```python
from build123d import *

# Parameters (mm, degrees)
SKETCH1_W           = 11
SKETCH1_H           = 70
SKETCH1_W_2         = 40
SKETCH1_H_2         = 18
BOSS_EXTRUDE1_DEPTH = 5
SKETCH3_W           = 23
SKETCH3_H           = 13
CUT_EXTRUDE2_DEPTH  = 57.868268832
SKETCH4_R           = 1.25
CUT_EXTRUDE3_DEPTH  = 57.868268832
SKETCH5_W           = 11
SKETCH5_H           = 75
BOSS_EXTRUDE2_DEPTH = 9
SKETCH6_W           = 3.5
SKETCH6_H           = 70
CUT_EXTRUDE4_DEPTH  = 59.352377844
SKETCH7_R           = 2
CUT_EXTRUDE5_DEPTH  = 61.458663564
RIB2_REACH          = 80.873
SKETCH8_WALL_W      = 176.81268046
SKETCH8_WALL_H      = 5
RIB4_REACH          = 80.873
SKETCH9_WALL_W      = 176.81268046
SKETCH9_WALL_H      = 5
RIB8_REACH          = 60.352
SKETCH10_WALL_W     = 139.567401732
SKETCH10_WALL_H     = 5
SKETCH14_W          = 42.5
SKETCH14_H          = 5
CUT_EXTRUDE6_DEPTH  = 61.458663564
CHAMFER9_SIZE       = 5
CHAMFER10_SIZE      = 2.5
CHAMFER11_SIZE      = 1
CHAMFER12_SIZE      = 1
SKETCH15_R          = 3.5
CUT_EXTRUDE7_DEPTH  = 2
CHAMFER14_SIZE      = 1


with BuildPart() as part:
    # Sketch1 → Boss-Extrude1 (new body)
    with BuildSketch(Plane(origin=(0, 0, 0), x_dir=(1, 0, 0), z_dir=(0, 1, 0))):
        Rectangle(SKETCH1_W, SKETCH1_H)
        with Locations((0, -44)):
            Rectangle(SKETCH1_W_2, SKETCH1_H_2)
    extrude(amount=BOSS_EXTRUDE1_DEPTH)

    # Sketch3 → Cut-Extrude2 (cut, through all)
    with BuildSketch(Plane(origin=(0, 5, 0), x_dir=(1, 0, 0), z_dir=(0, 1, 0))):
        with Locations((0, -46.5)):
            Rectangle(SKETCH3_W, SKETCH3_H)
    extrude(amount=-CUT_EXTRUDE2_DEPTH, mode=Mode.SUBTRACT)

    # Sketch4 → Cut-Extrude3 (cut, through all)
    with BuildSketch(Plane(origin=(0, 5, 0), x_dir=(1, 0, 0), z_dir=(0, 1, 0))):
        with Locations(Location((-13.5, -46.5, 0), (0, 0, 270))):
            Circle(SKETCH4_R)
        with Locations(Location((13.5, -46.5, 0), (0, 0, 270))):
            Circle(SKETCH4_R)
    extrude(amount=-CUT_EXTRUDE3_DEPTH, mode=Mode.SUBTRACT)

    # Sketch5 → Boss-Extrude2 (add)
    with BuildSketch(Plane(origin=(0, 5, 0), x_dir=(1, 0, 0), z_dir=(0, 1, 0))):
        with Locations((0, -2.5)):
            Rectangle(SKETCH5_W, SKETCH5_H)
    extrude(amount=BOSS_EXTRUDE2_DEPTH)

    # Sketch6 → Cut-Extrude4 (cut, through all)
    with BuildSketch(Plane.XZ):
        Rectangle(SKETCH6_W, SKETCH6_H)
    extrude(amount=-CUT_EXTRUDE4_DEPTH, mode=Mode.SUBTRACT)

    # Sketch7 → Cut-Extrude5 (cut, through all)
    with BuildSketch(Plane.ZY.offset(5.5)):
        with Locations((-28.5, 9.5)):
            Circle(SKETCH7_R)
        with Locations((30.5, 9.5)):
            Circle(SKETCH7_R)
    extrude(amount=-CUT_EXTRUDE5_DEPTH, mode=Mode.SUBTRACT)

    # Sketch8 wall → Rib2 (add, up to next)
    with BuildSketch(Plane(origin=(-12.75, 9.5, 40), x_dir=(-0.849640166198, -0.527362861778, 0), z_dir=(0.527362861778, -0.849640166198, 0)), mode=Mode.PRIVATE) as rib2_sk1:
        with Locations((0, 2.5)):
            Rectangle(SKETCH8_WALL_W, SKETCH8_WALL_H)
    rib2_tool1 = extrude(rib2_sk1.sketch, amount=RIB2_REACH, mode=Mode.PRIVATE) - part.part
    add(rib2_tool1.solids().sort_by_distance((-12.75, 9.5, 40))[0])

    # Sketch9 wall → Rib4 (add, up to next)
    with BuildSketch(Plane(origin=(12.75, 9.5, 40), x_dir=(0.849640166198, -0.527362861778, 0), z_dir=(0.527362861778, 0.849640166198, 0)), mode=Mode.PRIVATE) as rib4_sk1:
        with Locations((0, 2.5)):
            Rectangle(SKETCH9_WALL_W, SKETCH9_WALL_H)
    rib4_tool1 = extrude(rib4_sk1.sketch, amount=-RIB4_REACH, mode=Mode.PRIVATE) - part.part
    add(rib4_tool1.solids().sort_by_distance((12.75, 9.5, 40))[0])

    # Sketch10 wall → Rib8 (add, up to next)
    with BuildSketch(Plane(origin=(-12.75, 0, 27.5), x_dir=(0.695022096847, 0, -0.718988376049), z_dir=(0.718988376049, 0, 0.695022096847)), mode=Mode.PRIVATE) as rib8_sk1:
        with Locations((0, 2.5)):
            Rectangle(SKETCH10_WALL_W, SKETCH10_WALL_H)
    rib8_tool1 = extrude(rib8_sk1.sketch, amount=RIB8_REACH, mode=Mode.PRIVATE) - part.part
    rib8 = rib8_tool1.solids().sort_by_distance((-12.75, 0, 27.5))[0]
    add(rib8)

    # Mirror1: Rib8 across plane
    add(rib8.mirror(Plane(origin=(0, 0, 0), x_dir=(0, 0, 1), z_dir=(1, 0, 0))))

    # Sketch14 → Cut-Extrude6 (cut, through all)
    with BuildSketch(Plane(origin=(5.5, 0, 0), x_dir=(0, 0, -1), z_dir=(1, 0, 0))):
        with Locations((1.25, 11.5)):
            Rectangle(SKETCH14_W, SKETCH14_H)
    extrude(amount=-CUT_EXTRUDE6_DEPTH, mode=Mode.SUBTRACT)

    # Chamfer9
    chamfer9_edges = [part.edges().sort_by_distance(p)[0] for p in [
        (3.625, 9, -22.5),
        (-3.625, 9, -22.5),
        (3.625, 9, 20),
        (-3.625, 9, 20),
    ]]
    chamfer(chamfer9_edges, length=CHAMFER9_SIZE - 0.0001)  # a hair under: the kernel refuses the full size

    # Chamfer10
    chamfer10_edges = [part.edges().sort_by_distance(p)[0] for p in [
        (-3.625, 0, -35),
        (3.625, 14, -35),
        (-3.625, 14, -35),
        (3.625, 0, -35),
    ]]
    chamfer(chamfer10_edges, length=CHAMFER10_SIZE)

    # Chamfer11
    chamfer11_edges = [part.edges().sort_by_distance(p)[0] for p in [
        (-11.5, 2.5, 53),
        (11.5, 2.5, 53),
        (-20, 2.5, 53),
        (20, 2.5, 53),
    ]]
    chamfer(chamfer11_edges, length=CHAMFER11_SIZE)

    # Chamfer12
    chamfer12_edges = [part.edges().sort_by_distance(p)[0] for p in [
        (-11.5, 2.5, 40),
        (11.5, 2.5, 40),
    ]]
    chamfer(chamfer12_edges, length=CHAMFER12_SIZE)

    # Sketch15 → Cut-Extrude7 (cut)
    with BuildSketch(Plane(origin=(5.5, 0, 0), x_dir=(0, 0, -1), z_dir=(1, 0, 0))):
        with Locations((28.5, 9.5)):
            Circle(SKETCH15_R)
        with Locations((-30.5, 9.5)):
            Circle(SKETCH15_R)
    extrude(amount=-CUT_EXTRUDE7_DEPTH, mode=Mode.SUBTRACT)

    # Chamfer14
    chamfer14_edges = [part.edges().sort_by_distance(p)[0] for p in [
        (0, 14, 35),
        (0, 0, 35),
    ]]
    chamfer(chamfer14_edges, length=CHAMFER14_SIZE)


solid = part.part
```
Work out the finished part from the listing and answer in its coordinate system (mm). A direction names the side the tool comes from. Give positions to 0.01 mm unless a question says otherwise; leave off trailing zeros. Order: outer loops, then holes, each group sorted by start corner. A loop starts at its lowest first (then second) coordinate and runs counter-clockwise, first axis right, second up.
1. For faces 5 (the flat face through (9, 8, 35)), 6 (the cylindrical face through (4.514, 6.395, 28.885)), 7 (the flat face through (-16, 5, 46)), determine the directions among +Z, -Z, +X, -X, +Y, -Y from which every point of the face is accessible in a straight line to the end or side of a thin tool.
Result sheet:
face 5: -Z, +X, +Y
face 6: +X
face 7: +Z, +X, -X, +Y
2. Straight lines are drawn through the part: L1, parallel to X at y = 1.75, z = 46.5; L2, parallel to X at y = 0.75, z = -3. For each, find the intervals that lie inside material, in ascending order.
Result sheet:
L1: x = -20 to -14.75, -12.25 to -11.5, 11.5 to 12.25, 14.75 to 20
L2: x = -5.5 to -1.75, 1.75 to 5.5
3. Section A-A, the plane z = -28.5 is taken. Determine the outline of the cut face in (x, y).
Result sheet:
outline: (-5.5, 0) - (-1.75, 0) - (-1.75, 7.5) - (-5.5, 7.5) - close; (-5.5, 11.5) - (-1.75, 11.5) - (-1.75, 14) - (-5.5, 14) - close; (1.75, 0) - (5.5, 0) - (5.5, 6) - (3.5, 6) - (3.5, 7.5) - (1.75, 7.5) - close; (1.75, 11.5) - (3.5, 11.5) - (3.5, 13) - (5.5, 13) - (5.5, 14) - (1.75, 14) - close
4. The mould has two halves that part along Z. Classify faces 1 (the flat face through (4, 9, -1)), 2 (the flat face through (1, 7, 40)), 3 (the flat face through (0, 7, 35)), 4 (the flat face through (16, 5, 46)): released by +Z, released by -Z, zero draft, split by the parting line, or undercut.
Result sheet:
face 1: undercut
face 2: released by +Z
face 3: released by -Z
face 4: zero draft
5. Section D-D, the plane x = 0 is taken. Determine the outline of the cut face in (y, z).
Result sheet:
outline: (0, 36) - (1, 35) - (13, 35) - (14, 36) - (14, 40) - (0, 40) - close
6. Section C-C, the plane y = 4 is taken. Determine the outline of the cut face in (x, z).
Result sheet:
outline: (-20, 35) - (-5.5, 20) - (-5.5, -35) - (-1.75, -35) - (-1.75, 35) - (1.75, 35) - (1.75, -35) - (5.5, -35) - (5.5, 20) - (20, 35) - (20, 52) - (19, 53) - (12.5, 53) - (11.5, 52) - (11.5, 41) - (10.5, 40) - (-10.5, 40) - (-11.5, 41) - (-11.5, 52) - (-12.5, 53) - (-19, 53) - (-20, 52) - close; hole circle Ø2.5 at (-13.5, 46.5); hole circle Ø2.5 at (13.5, 46.5)
7. Each of these flat-tipped pins is pushed along its axis until it touches: P1, Ø4.5, axis at x = 12, y = 8.5, coming from the -Z side; P2, Ø6, axis at y = 10.5, z = 7, coming from the +X side; P3, Ø4, axis at x = -7.5, y = 6.5, coming from the +Z side. Where does it stop, or does it pass through?
Result sheet:
P1: stops at z = 35
P2: stops at x = 5.5
P3: stops at z = 40
8. Section B-B, the plane z = -9.5 is taken. Determine the outline of the cut face in (x, y).
Result sheet:
outline: (-5.5, 0) - (-1.75, 0) - (-1.75, 9) - (-5.5, 9) - close; (1.75, 0) - (5.5, 0) - (5.5, 9) - (1.75, 9) - close
